```python
from build123d import *

# Parameters (mm, degrees)
EXTRUDE_1_DEPTH     = 80
FILLET_1_R          = 2
SKETCH_2_R          = 1
CUT_EXTRUDE_1_DEPTH = 5


with BuildPart() as part:
    # 草图1 → 凸台-拉伸1 (new body)
    with BuildSketch(Plane(origin=(0, 0, 0), x_dir=(0, 0, -1), z_dir=(1, 0, 0))):
        with BuildLine():
            Line((-30, 0), (30, 0))
            Line((30, 0), (30, 15))
            ThreePointArc((30, 15), (0, 8.245553203), (-30, 15))
            Line((-30, 15), (-30, 0))
        make_face()
    extrude(amount=EXTRUDE_1_DEPTH)

    # 圆角1
    fillet_1_edges = [part.edges().sort_by_distance(p)[0] for p in [
        (40, 15, 30),
        (40, 15, -30),
    ]]
    fillet(fillet_1_edges, radius=FILLET_1_R)

    # 草图2 → 切除-拉伸1 (cut)
    with BuildSketch(Plane(origin=(80, 0, 0), x_dir=(0, 0, -1), z_dir=(1, 0, 0))):
        with Locations((-25, 7.5)):
            Circle(SKETCH_2_R)
        with Locations((25, 7.5)):
            Circle(SKETCH_2_R)
    cut_extrude_1 = extrude(amount=-CUT_EXTRUDE_1_DEPTH, mode=Mode.SUBTRACT)

    # 镜向1: 切除-拉伸1 across plane
    add(cut_extrude_1.mirror(Plane(origin=(40, 0, 0), x_dir=(0, 0, 1), z_dir=(1, 0, 0))), mode=Mode.SUBTRACT)


solid = part.part
```
Work out the finished part from the listing and answer in its coordinate system (mm). A direction names the side the tool comes from. Give positions to 0.01 mm unless a question says otherwise; leave off trailing zeros. Order: outer loops, then holes, each group sorted by start corner. A loop starts at its lowest first (then second) coordinate and runs counter-clockwise, first axis right, second up.
1. Section A-A, the plane y = 10 is taken. Determine the outline of the cut face in (x, z).
Result sheet:
outline: (0, -30) - (80, -30) - (80, -15.57) - (0, -15.57) - close; (0, 15.57) - (80, 15.57) - (80, 30) - (0, 30) - close
2. Straight lines are drawn through the part: L1, parallel to Y at x = 56, z = -6; L2, parallel to Y at x = 77.45, z = -25; L3, parallel to Y at x = 64.5, z = 23.5. For each, find the intervals that lie inside material, in ascending order.
Result sheet:
L1: y = 0 to 8.5
L2: y = 0 to 6.5, 8.5 to 12.86
L3: y = 0 to 12.31
3. Each of these flat-tipped pins is pushed along its axis until it touches: P1, Ø1.2, axis at y = 7.5, z = 25, coming from the +X side; P2, Ø3, axis at x = 25, z = -23, coming from the +Y side; P3, Ø6, axis at x = 35, z = -13, coming from the +Y side. Where does it stop, or does it pass through?
Result sheet:
P1: stops at x = 75
P2: stops at y = 12.67
P3: stops at y = 10.1
4. Section B-B, the plane z = 25 is taken. Determine the outline of the cut face in (x, y).
Result sheet:
outline: (0, 0) - (80, 0) - (80, 6.5) - (75, 6.5) - (75, 8.5) - (80, 8.5) - (80, 12.86) - (0, 12.86) - (0, 8.5) - (5, 8.5) - (5, 6.5) - (0, 6.5) - close
5. Section C-C, the plane x = 34 is taken. Determine the outline of the cut face in (y, z).
Result sheet:
outline: (0, -30) - (11.91, -30) arc R2 ccw to (13.76, -27.22) arc R70 cw to (13.76, 27.22) arc R2 ccw to (11.91, 30) - (0, 30) - close
6. For faces 4 (the flat face through (75, 8, 25)), 5 (the cylindrical face through (40.56, 13.595, 29.082)), 6 (the cylindrical face through (2.465, 7.8, -25.954)), determine the directions among +Z, -Z, +X, -X, +Y, -Y from which every point of the face is accessible in a straight line to the end or side of a thin tool.
Result sheet:
face 4: +X
face 5: +X, -X, +Y
face 6: -X
7. The mould has two halves that part along Y. Classify faces 1 (the cylindrical face through (2.46, 8.49, 25.13)), 2 (the cylindrical face through (40.56, 13.564, -29.128)), 3 (the flat face through (39, 6, 30)): released by +Y, released by -Y, zero draft, split by the parting line, or undercut.
Result sheet:
face 1: undercut
face 2: released by +Y
face 3: zero draft
8. Section D-D, the plane z = -2 is taken. Determine the outline of the cut face in (x, y), and give its area (3 significant figures).
Result sheet:
outline: (0, 0) - (80, 0) - (80, 8.27) - (0, 8.27) - close
area: 662 mm2
